Print and shaded views of the part. All mm, measured from the part's lowest x, y and z. Coordinates: 2 decimals unless noted, no trailing zeros. Loops run counter-clockwise (first coordinate to the right, second up) from the corner with the lowest first, then second, coordinate; pieces in that order, holes last. Notation, with made-up numbers: M 49.25,77 L 79.25,77 A24 ccw 79.25,113 Z; hole C 75.5,55.25 d2. An arc over 180 degrees is marked long. Use a Markdown table: item, result. Add a question column.
1) Band-saw the part on A-A (y = 4). List the corners of the cut face in (x, z).
2) Wall check: probe 1 along Z at (x, y) = (0.75, 1); probe 2 along X at (y, z) = (1.75, 1.2); probe 3 along Y at (x, z) = (13, 0.5). Give the ranges that are in metal, low to high. Write a range as from..to.
3) Pin check, flat tip, straight feed: pin 1 Ø1 at (y, z) = (8, 0.5) entering from +X. Stop position of the tip, or through.
4) Band-saw the part on B-B (x = 17). List the corners of the cut face in (y, z), plus the area to 3 significant figures.
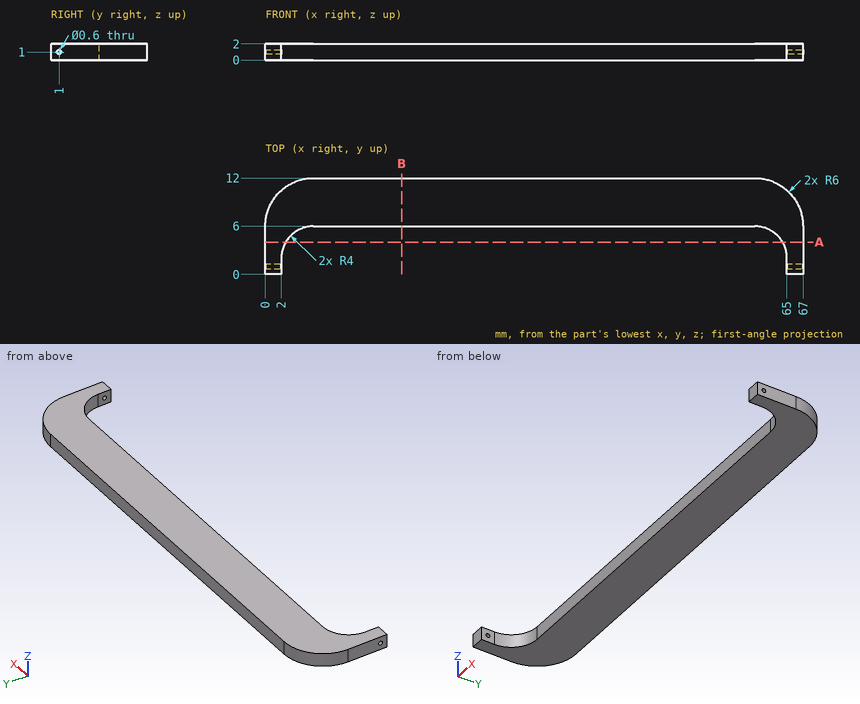
Entries:
| question | item | result |
|---|---|---|
| 1 | outline | M 0,0 L 2.54,0 L 2.54,2 L 0,2 Z; M 64.46,0 L 67,0 L 67,2 L 64.46,2 Z |
| 2 | probe 1 | 0..0.7, 1.3..2 |
| 2 | probe 2 | 0..2, 65..67 |
| 2 | probe 3 | 6..12 |
| 3 | pin 1 | x = 66.81 |
| 4 | outline | M 6,0 L 12,0 L 12,2 L 6,2 Z |
| 4 | area | 12.0 mm2 |
